For this review, take the finished solid that the model builds, in its own axes (mm). A direction names the side the tool comes from. Give positions to 0.01 mm unless a question says otherwise; leave off trailing zeros. Order: outer loops, then holes, each group sorted by start corner. A loop starts at its lowest first (then second) coordinate and runs counter-clockwise, first axis right, second up. Notation, with made-up numbers: (89.25, 77.5) -> (148.25, 77.5) arc R24 cw to (148.25, 95.5) -> close; hole circle Ø6 at (57.25, 74). An arc over 180 degrees is marked (long way). Return JSON: item names as keys, results as strings. Group by question number.
1) Add section A-A (y = 15). Give the boundary of the cut face in (x, z).
2) For faces 1 (the face through (66, 24, 20)), 2 (the face through (100, 8, 33)), 3 (the face through (59, -5, 55)), 4 (the face through (0, 35, 48)), 5 (the face through (32, -10, 15)), list the 3-axis set-ups (+Z, -Z, +X, -X, +Y, -Y) from which the entire face can be reached by the end or side of a thin tool; tool diameter is ignored.
3) Insertion check: P1, Ø8, axis at x = 55, y = 6, coming from the +Z side; P2, Ø5, axis at y = 34.5, z = 51, coming from the -X side; P3, Ø4, axis at x = 99, z = 35, coming from the -Y side; P4, Ø15, axis at y = 21, z = 21.5, coming from the +X side. Each pin has a flat end and moves straight along its axis. Give the tip position at first contact, or say it passes through.
4) Add section C-C (z = 4). Give the boundary of the cut face in (x, y), then the cut area to 3 significant figures.
5) The part is to be moulded in two halves that separate along Y. For faces 6 (the face through (37, 15, 0)), 7 (the face through (119, -1, 41)), 8 (the face through (32, 40, 15)), say which applies: released by +Y, released by -Y, zero draft, split by the parting line, or undercut.
6) To check wall thickness, follow line 1 along X through (y, z) = (9, 19.5); line 2 along X through (y, z) = (2, 31.5); line 3 along Y through (x, z) = (71.5, 11). State the ranges of each line that lie inside material, in increasing order.
7) Add section D-D (x = 43). Give the boundary of the cut face in (y, z).
8) Add section B-B (z = 50). Give the boundary of the cut face in (x, y).
from build123d import *

# Parameters (mm, degrees)
BOX051_W          = 10
BOX051_H          = 8
BOX051_DEPTH      = 40
BOX050_W          = 67
BOX050_H          = 14
BOX050_DEPTH      = 25
BOX049_W          = 67
BOX049_H          = 30
BOX049_DEPTH      = 15
BOX048_W          = 119
BOX048_H          = 70
BOX048_DEPTH      = 30
BOX046_W          = 66
BOX046_H          = 30
BOX046_DEPTH      = 60
CYLINDER101_R     = 25
CYLINDER101_DEPTH = 119
BOX047_W          = 86
BOX047_H          = 50
BOX047_DEPTH      = 50


with BuildPart() as cube030:
    # Box051 → Box051 (new body)
    with BuildSketch(Plane(origin=(66, 11, 0), x_dir=(1, 0, 0), z_dir=(0, 0, 1))):
        with Locations((5, 4)):
            Rectangle(BOX051_W, BOX051_H)
    extrude(amount=BOX051_DEPTH)


with BuildPart() as cube029:
    # Box050 → Box050 (new body)
    with BuildSketch(Plane(origin=(81, 8, 15), x_dir=(1, 0, 0), z_dir=(0, 0, 1))):
        with Locations((33.5, 7)):
            Rectangle(BOX050_W, BOX050_H)
    extrude(amount=BOX050_DEPTH)


with BuildPart() as cube028:
    # Box049 → Box049 (new body)
    with BuildSketch(Plane(origin=(66, 0, 40), x_dir=(1, 0, 0), z_dir=(0, 0, 1))):
        with Locations((33.5, 15)):
            Rectangle(BOX049_W, BOX049_H)
    extrude(amount=BOX049_DEPTH)


with BuildPart() as cube027:
    # Box048 → Box048 (new body)
    with BuildSketch(Plane(origin=(0, -13, 55), x_dir=(1, 0, 0), z_dir=(0, 0, 1))):
        with Locations((59.5, 35)):
            Rectangle(BOX048_W, BOX048_H)
    extrude(amount=BOX048_DEPTH)


with BuildPart() as cube025:
    # Box046 → Box046 (new body)
    with BuildSketch(Plane.XY):
        with Locations((33, 15)):
            Rectangle(BOX046_W, BOX046_H)
    extrude(amount=BOX046_DEPTH)


with BuildPart() as cut111:
    # Cylinder101 → Cylinder101 (new body)
    with BuildSketch(Plane(origin=(0, 15, 50), x_dir=(0, 0, -1), z_dir=(1, 0, 0))):
        Circle(CYLINDER101_R)
    extrude(amount=CYLINDER101_DEPTH)

    # Cut108: cut Cube025
    add(cube025.part, mode=Mode.SUBTRACT)

    # Cut109: cut Cube027
    add(cube027.part, mode=Mode.SUBTRACT)

    # Cut110: cut Cube028
    add(cube028.part, mode=Mode.SUBTRACT)

    # Cut111: cut Cube029
    add(cube029.part, mode=Mode.SUBTRACT)


with BuildPart() as cut112:
    # Box047 → Box047 (new body)
    with BuildSketch(Plane(origin=(-10, -10, -10), x_dir=(1, 0, 0), z_dir=(0, 0, 1))):
        with Locations((43, 25)):
            Rectangle(BOX047_W, BOX047_H)
    extrude(amount=BOX047_DEPTH)

    # Cut107: cut Cube025
    add(cube025.part, mode=Mode.SUBTRACT)

    # Fusion031: union Cut111
    add(cut111.part)

    # Cut112: cut Cube030
    add(cube030.part, mode=Mode.SUBTRACT)


solid = cut112.part
Evaluation:
{
 "1": {"outline": "(-10, -10) -> (76, -10) -> (76, 0) -> (0, 0) -> (0, 40) -> (-10, 40) -> close; (76, 25) -> (81, 25) -> (81, 40) -> (76, 40) -> close"},
 "2": {"face 1": "+Z", "face 2": "+Z, -Z, +X", "face 3": "+Z, +X, -X, +Y, -Y", "face 4": "+Z, -X, +Y, -Y", "face 5": "+Z, -Z, +X, -X, -Y"},
 "3": {"P1": "z = 0", "P2": "x = 0", "P3": "y = -6.35", "P4": "x = 119"},
 "4": {"outline": "(-10, -10) -> (76, -10) -> (76, 11) -> (66, 11) -> (66, 0) -> (0, 0) -> (0, 30) -> (66, 30) -> (66, 19) -> (76, 19) -> (76, 40) -> (-10, 40) -> close", "area": "2,240 mm^2"},
 "5": {"face 6": "undercut", "face 7": "zero draft", "face 8": "released by +Y"},
 "6": {"line 1": "-10 to 0, 66 to 76", "line 2": "-10 to 0, 66 to 119", "line 3": "-10 to 11, 19 to 40"},
 "7": {"outline": "(-10, -10) -> (40, -10) -> (40, 40) -> (37.91, 40) arc R25 ccw to (39.49, 55) -> (30, 55) -> (30, 0) -> (0, 0) -> (0, 55) -> (-9.49, 55) arc R25 ccw to (-7.91, 40) -> (-10, 40) -> close"},
 "8": {"outline": "(0, -10) -> (119, -10) -> (119, 0) -> (0, 0) -> close; (0, 30) -> (119, 30) -> (119, 40) -> (0, 40) -> close"}
}
